Model file for the job. Use its own axes, mm. A direction names the side the tool comes from. Give positions to 0.01 mm unless a question says otherwise; leave off trailing zeros. Write each loop counter-clockwise with the first axis right and the second up, starting at its lowest first coordinate (ties: lowest second). Pieces come first, ordered by that corner, then holes.
```python
from build123d import *

# Parameters (mm, degrees)
BOSS_EXTRUDE1_DEPTH = 10


with BuildPart() as part:
    # Sketch1 → Boss-Extrude1 (new body)
    with BuildSketch(Plane(origin=(0, 0, 0), x_dir=(1, 0, 0), z_dir=(0, 1, 0))):
        with BuildLine():
            Line((7.002608144, 23.999239138), (0, 34))
            Line((0, 34), (-7.002608144, 23.999239138))
            ThreePointArc((-7.002608144, 23.999239138), (-9.567085809, 23.096988313), (-12.018433033, 21.921616442))
            Line((-12.018433033, 21.921616442), (-24.04163056, 24.04163056))
            Line((-24.04163056, 24.04163056), (-21.921616442, 12.018433033))
            ThreePointArc((-21.921616442, 12.018433033), (-23.096988313, 9.567085809), (-23.999239138, 7.002608144))
            Line((-23.999239138, 7.002608144), (-34, 0))
            Line((-34, 0), (-23.999239138, -7.002608144))
            ThreePointArc((-23.999239138, -7.002608144), (-23.096988313, -9.567085809), (-21.921616442, -12.018433033))
            Line((-21.921616442, -12.018433033), (-24.04163056, -24.04163056))
            Line((-24.04163056, -24.04163056), (-12.018433033, -21.921616442))
            ThreePointArc((-12.018433033, -21.921616442), (-9.567085809, -23.096988313), (-7.002608144, -23.999239138))
            Line((-7.002608144, -23.999239138), (0, -34))
            Line((0, -34), (7.002608144, -23.999239138))
            ThreePointArc((7.002608144, -23.999239138), (9.567085809, -23.096988313), (12.018433033, -21.921616442))
            Line((12.018433033, -21.921616442), (24.04163056, -24.04163056))
            Line((24.04163056, -24.04163056), (21.921616442, -12.018433033))
            ThreePointArc((21.921616442, -12.018433033), (23.096988313, -9.567085809), (23.999239138, -7.002608144))
            Line((23.999239138, -7.002608144), (34, 0))
            Line((34, 0), (23.999239138, 7.002608144))
            ThreePointArc((23.999239138, 7.002608144), (23.096988313, 9.567085809), (21.921616442, 12.018433033))
            Line((21.921616442, 12.018433033), (24.04163056, 24.04163056))
            Line((24.04163056, 24.04163056), (12.018433033, 21.921616442))
            ThreePointArc((12.018433033, 21.921616442), (9.567085809, 23.096988313), (7.002608144, 23.999239138))
        make_face()
    extrude(amount=BOSS_EXTRUDE1_DEPTH)


solid = part.part
```
1. Slice it at C-C, the plane z = -16. Write the cut outline in (x, y), and give its area (3 significant figures).
Calculated:
outline: (-22.62, 0) - (22.62, 0) - (22.62, 10) - (-22.62, 10) - close
area: 452 mm2
2. Probe probe 1 along Z at (x, y) = (11.5, 9.25); probe 2 along Z at (x, y) = (11, 6); probe 3 along X at (y, z) = (3.75, -25). List the from-to ranges inside material, lowest first.
Calculated:
probe 1: z = -22.2 to 22.2
probe 2: z = -22.45 to 22.45
probe 3: x = -6.3 to 6.3
3. Slice it at B-B, the plane x = 5. Write the cut outline in (y, z), and give its area (3 significant figures).
Calculated:
outline: (0, -26.86) - (10, -26.86) - (10, 26.86) - (0, 26.86) - close
area: 537 mm2
4. Which spindle directions (+Z, -Z, +X, -X, +Y, -Y) get a long thin tool onto all of the face, cutting with end or side? Do faces 5 (the cylindrical face through (-23.082, 4.93, -9.602)), 6 (the cylindrical face through (23.082, 4.93, 9.602)), 7 (the cylindrical face through (9.602, 4.93, -23.082)). Say none if no direction does.
Calculated:
face 5: -X, +Y, -Y
face 6: +X, +Y, -Y
face 7: -Z, +Y, -Y
5. Pull direction X, two halves, no side cores. Call faces 1 (the cylindrical face through (9.532, 4.93, 23.112)), 2 (the flat face through (-22.996, 4.93, -18.114)), 3 (the flat face through (18.114, 4.93, -22.996)), 4 (the flat face through (22.967, 4.93, -17.946)): +X half, -X half, draft (parallel to the pull), parting line (faces both ways), or undercut.
Calculated:
face 1: undercut
face 2: -X half
face 3: undercut
face 4: +X half
6. Pin check, flat tips, straight feed: P1, Ø2, axis at x = 16.5, y = 1, coming from the +Z side; P2, Ø4, axis at y = 5, z = -18, coming from the -X side; P3, Ø2, axis at x = 9.5, y = 3, coming from the -Z side; P4, Ø5, axis at x = 11, z = 25.5, coming from the +Y side. Stop position of each tip, or through.
Calculated:
P1: stops at z = 22.89
P2: stops at x = -23.33
P3: stops at z = -23.51
P4: passes through
7. Slice it at A-A, the plane y = 9. Write the cut outline in (x, z), and give its area (3 significant figures).
Calculated:
outline: (-34, 0) - (-24, -7) arc R25 ccw to (-21.92, -12.02) - (-24.04, -24.04) - (-12.02, -21.92) arc R25 ccw to (-7, -24) - (0, -34) - (7, -24) arc R25 ccw to (12.02, -21.92) - (24.04, -24.04) - (21.92, -12.02) arc R25 ccw to (24, -7) - (34, 0) - (24, 7) arc R25 ccw to (21.92, 12.02) - (24.04, 24.04) - (12.02, 21.92) arc R25 ccw to (7, 24) - (0, 34) - (-7, 24) arc R25 ccw to (-12.02, 21.92) - (-24.04, 24.04) - (-21.92, 12.02) arc R25 ccw to (-24, 7) - close
area: 2,450 mm2
